The listing builds one solid part. Answer for the finished solid, in the listing's coordinates (mm). A direction names the side the tool comes from. Give positions to 0.01 mm unless a question says otherwise; leave off trailing zeros. Order: outer loops, then holes, each group sorted by start corner. A loop starts at its lowest first (then second) coordinate and runs counter-clockwise, first axis right, second up.
```python
from build123d import *

# Parameters (mm, degrees)
SKIZZE2_W                       = 310
SKIZZE2_H                       = 50
AUFSATZ_LINEAR_AUSTRAGEN1_DEPTH = 85
SKIZZE4_W                       = 290
SKIZZE4_H                       = 65
SCHNITT_LINEAR_AUSTRAGEN1_DEPTH = 30
VERRUNDUNG1_R                   = 10
VERRUNDUNG2_R                   = 10
VERRUNDUNG3_R                   = 10
VERRUNDUNG4_R                   = 10
SKIZZE9_W                       = 8
SKIZZE9_H                       = 4
SCHNITT_LINEAR_AUSTRAGEN2_DEPTH = 10
SKIZZE10_R                      = 1.5
SCHNITT_LINEAR_AUSTRAGEN3_DEPTH = 6


with BuildPart() as part:
    # Skizze2 → Aufsatz-Linear austragen1 (new body)
    with BuildSketch(Plane.XY):
        with Locations((155, 25)):
            Rectangle(SKIZZE2_W, SKIZZE2_H)
    extrude(amount=AUFSATZ_LINEAR_AUSTRAGEN1_DEPTH)

    # Skizze4 → Schnitt-Linear austragen1 (cut)
    with BuildSketch(Plane(origin=(0, 50, 0), x_dir=(1, 0, 0), z_dir=(0, 1, 0))):
        with Locations((155, -42.5)):
            Rectangle(SKIZZE4_W, SKIZZE4_H)
    extrude(amount=-SCHNITT_LINEAR_AUSTRAGEN1_DEPTH, mode=Mode.SUBTRACT)

    # Verrundung1
    verrundung1_edges = [part.edges().sort_by_distance(p)[0] for p in [
        (310, 25, 0),
    ]]
    fillet(verrundung1_edges, radius=VERRUNDUNG1_R)

    # Verrundung2
    verrundung2_edges = [part.edges().sort_by_distance(p)[0] for p in [
        (310, 25, 85),
    ]]
    fillet(verrundung2_edges, radius=VERRUNDUNG2_R)

    # Verrundung3
    verrundung3_edges = [part.edges().sort_by_distance(p)[0] for p in [
        (0, 25, 85),
    ]]
    fillet(verrundung3_edges, radius=VERRUNDUNG3_R)

    # Verrundung4
    verrundung4_edges = [part.edges().sort_by_distance(p)[0] for p in [
        (0, 25, 0),
    ]]
    fillet(verrundung4_edges, radius=VERRUNDUNG4_R)

    # Skizze9 → Schnitt-Linear austragen2 (cut)
    with BuildSketch(Plane(origin=(0, 0, 0), x_dir=(-1, 0, 0), z_dir=(0, 0, -1))):
        with Locations((-286, 27)):
            Rectangle(SKIZZE9_W, SKIZZE9_H)
    extrude(amount=-SCHNITT_LINEAR_AUSTRAGEN2_DEPTH, mode=Mode.SUBTRACT)

    # Skizze10 → Schnitt-Linear austragen3 (cut)
    with BuildSketch(Plane(origin=(0, 20, 0), x_dir=(1, 0, 0), z_dir=(0, 1, 0))):
        with Locations(Location((286, -15, 0), (0, 0, 270))):
            Circle(SKIZZE10_R)
        with Locations(Location((286, -70, 0), (0, 0, 270))):
            Circle(SKIZZE10_R)
    extrude(amount=-SCHNITT_LINEAR_AUSTRAGEN3_DEPTH, mode=Mode.SUBTRACT)


solid = part.part
```
1) For a pull along X with two mould halves and no side action, classify faces 4 (the flat face through (310, 25, 42)), 5 (the flat face through (143, 50, 77)), 6 (the flat face through (153, 35, 75)) as +X half, -X half, draft (parallel to the pull), parting line (faces both ways), or undercut.
Geometry says:
face 4: +X half
face 5: draft
face 6: undercut
2) Find section A-A (z = 65.5). Write down the section's boundary in (x, y).
Geometry says:
outline: (0, 0) - (310, 0) - (310, 50) - (300, 50) - (300, 20) - (10, 20) - (10, 50) - (0, 50) - close
3) Given P1, Ø0.9, axis at x = 286, z = 15.5, coming from the +Y side; P2, Ø2.5, axis at x = 286.5, z = 70, coming from the +Y side; P3, Ø1.2, axis at y = 28, z = 6.5, coming from the +X side, each flat-ended and moving along its own axis, determine where each tip first touches the part or whether it passes through.
Geometry says:
P1: stops at y = 14
P2: stops at y = 20
P3: stops at x = 309.57
4) A tool of negligible diameter and unlimited length cuts with its end or side. For faces 1 (the flat face through (153, 20, 42)), 2 (the flat face through (0, 25, 42)), 3 (the flat face through (286, 29, 5)), from which of +Z, -Z, +X, -X, +Y, -Y can it reach the whole face along a straight path? Write none if from no direction.
Geometry says:
face 1: +Y
face 2: +Z, -Z, -X, +Y, -Y
face 3: -Z
5) Straight lines are drawn through the part: probe 1 along Z at (x, y) = (286, 16); probe 2 along X at (y, z) = (18.5, 70); probe 3 along Z at (x, y) = (88.5, 39). For each, find the intervals that lie inside material, in ascending order.
Geometry says:
probe 1: z = 0 to 13.5, 16.5 to 68.5, 71.5 to 85
probe 2: x = 0 to 284.5, 287.5 to 310
probe 3: z = 0 to 10, 75 to 85
6) Find section B-B (x = 235). Write down the section's boundary in (y, z), then the cut area to 3 significant figures.
Geometry says:
outline: (0, 0) - (50, 0) - (50, 10) - (20, 10) - (20, 75) - (50, 75) - (50, 85) - (0, 85) - close
area: 2,300 mm2
